from build123d import *

# Parameters (mm, degrees)
SKETCH1_R           = 40
BOSS_EXTRUDE1_DEPTH = 4
SKETCH2_R           = 25
BOSS_EXTRUDE2_DEPTH = 6
SKETCH3_R           = 1.5
CUT_EXTRUDE1_DEPTH  = 5
SKETCH4_R           = 9
CUT_EXTRUDE2_DEPTH  = 58.445626465
SKETCH5_R           = 1.5
CUT_EXTRUDE3_DEPTH  = 57.789083458
SKETCH6_R           = 2.84
CUT_EXTRUDE4_DEPTH  = 3


with BuildPart() as part:
    # Sketch1 → Boss-Extrude1 (new body)
    with BuildSketch(Plane(origin=(0, 0, 0), x_dir=(1, 0, 0), z_dir=(0, 1, 0))):
        with Locations(Location((0, 0, 0), (0, 0, 270))):
            Circle(SKETCH1_R)
    extrude(amount=BOSS_EXTRUDE1_DEPTH)

    # Sketch2 → Boss-Extrude2 (add)
    with BuildSketch(Plane(origin=(0, 4, 0), x_dir=(1, 0, 0), z_dir=(0, 1, 0))):
        with Locations(Location((0, 0, 0), (0, 0, 270))):
            Circle(SKETCH2_R)
    extrude(amount=BOSS_EXTRUDE2_DEPTH)

    # Sketch3 → Cut-Extrude1 (cut)
    with BuildSketch(Plane(origin=(0, 10, 0), x_dir=(1, 0, 0), z_dir=(0, 1, 0))):
        with Locations(Location((0, -21.5, 0), (0, 0, 270))):
            Circle(SKETCH3_R)
        with Locations(Location((-15.202795796, -15.202795796, 0), (0, 0, 270))):
            Circle(SKETCH3_R)
        with Locations(Location((-21.5, 0, 0), (0, 0, 270))):
            Circle(SKETCH3_R)
        with Locations(Location((-15.202795796, 15.202795796, 0), (0, 0, 270))):
            Circle(SKETCH3_R)
        with Locations(Location((0, 21.5, 0), (0, 0, 270))):
            Circle(SKETCH3_R)
        with Locations(Location((15.202795796, 15.202795796, 0), (0, 0, 270))):
            Circle(SKETCH3_R)
        with Locations(Location((21.5, 0, 0), (0, 0, 270))):
            Circle(SKETCH3_R)
        with Locations(Location((15.202795796, -15.202795796, 0), (0, 0, 270))):
            Circle(SKETCH3_R)
    extrude(amount=-CUT_EXTRUDE1_DEPTH, mode=Mode.SUBTRACT)

    # Sketch4 → Cut-Extrude2 (cut, through all)
    with BuildSketch(Plane(origin=(0, 10, 0), x_dir=(1, 0, 0), z_dir=(0, 1, 0))):
        with Locations(Location((0, 0, 0), (0, 0, 270))):
            Circle(SKETCH4_R)
    extrude(amount=-CUT_EXTRUDE2_DEPTH, mode=Mode.SUBTRACT)

    # Sketch5 → Cut-Extrude3 (cut, through all)
    with BuildSketch(Plane(origin=(0, 5, 0), x_dir=(1, 0, 0), z_dir=(0, 1, 0))):
        with Locations(Location((15.202795796, 15.202795796, 0), (0, 0, 270))):
            Circle(SKETCH5_R)
        with Locations(Location((-15.202795796, -15.202795796, 0), (0, 0, 270))):
            Circle(SKETCH5_R)
    extrude(amount=-CUT_EXTRUDE3_DEPTH, mode=Mode.SUBTRACT)

    # Sketch6 → Cut-Extrude4 (cut)
    with BuildSketch(Plane.XZ):
        with Locations(Location((-15.202795796, 15.202795796, 0), (0, 0, 270))):
            Circle(SKETCH6_R)
        with Locations(Location((15.202795796, -15.202795796, 0), (0, 0, 270))):
            Circle(SKETCH6_R)
    extrude(amount=-CUT_EXTRUDE4_DEPTH, mode=Mode.SUBTRACT)


solid = part.part
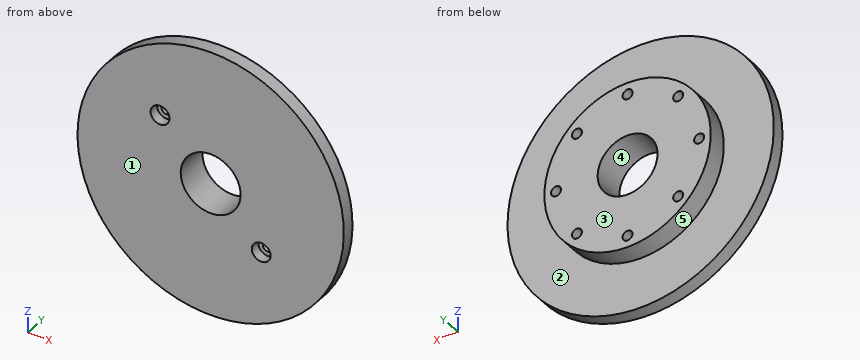
Here's how the part is built. I have some questions about the finished solid (model axes, mm). Face numbers are marked on the shaded views. A direction names the side the tool comes from. Round coordinates to 2 decimals unless told otherwise and drop trailing zeros. Write each loop counter-clockwise with the first axis right and the second up, starting at its lowest first coordinate (ties: lowest second). Pieces come first, ordered by that corner, then holes.
1. Will these pins go through, and if not, where does the flat tip stop? pin 1 Ø1.5 at (y, z) = (4, -3) entering from -X; pin 2 Ø5 at (y, z) = (4, 1) entering from -X; pin 3 Ø1.5 at (x, z) = (0.5, -21.5) entering from +Y.
2. For the marked faces 1 and 2, which set-ups out of +Z, -Z, +X, -X, +Y, -Y let a thin tool reach every point of the face, with its end or its side?
3. If we mould it in two halves opening along X, with no side actions, what happens to the marked faces 3, 4 and 5? For each: released by +X, released by -X, zero draft, split by the parting line, or undercut.
4. I need wall thicknesses on L1, parallel to Y at x = -10, z = -26.5; L2, parallel to Z at x = -8, y = 6.25; L3, parallel to Z at x = -4.5, y = 5.25. Which ranges of each line are inside material? Lowest first, please.
5. Suppose I cut it at B-B (z = -6.5). List the corners of the cut face in (x, y) for me.
6. Suppose I cut it at C-C (y = 8). State how many separate pieces and enclosed holes the cut face has, and give its area (3 significant figures).
7. Suppose I cut it at A-A (x = 0). List the corners of the cut face in (y, z) for me.
8. Suppose I cut it at D-D (x = 19). List the corners of the cut face in (y, z) for me.
Answer sheet:
1. pin 1: stops at x = -39.94
1. pin 2: stops at x = -40
1. pin 3: stops at y = 5
2. face 1: +Z, -Z, +X, -X, -Y
2. face 2: +Y
3. face 3: zero draft
3. face 4: undercut
3. face 5: split by the parting line
4. L1: y = 0 to 4
4. L2: z = -23.69 to -4.12, 4.12 to 23.69
4. L3: z = -24.59 to -7.79, 7.79 to 24.59
5. outline: (-39.47, 0) - (-6.22, 0) - (-6.22, 10) - (-24.14, 10) - (-24.14, 4) - (-39.47, 4) - close; (6.22, 0) - (39.47, 0) - (39.47, 4) - (24.14, 4) - (24.14, 10) - (6.22, 10) - close
6. separate pieces: 1
6. enclosed holes: 9
6. area: 1,650 mm2
7. outline: (0, -40) - (4, -40) - (4, -25) - (10, -25) - (10, -23) - (5, -23) - (5, -20) - (10, -20) - (10, -9) - (0, -9) - close; (0, 9) - (10, 9) - (10, 20) - (5, 20) - (5, 23) - (10, 23) - (10, 25) - (4, 25) - (4, 40) - (0, 40) - close
8. outline: (0, -35.2) - (4, -35.2) - (4, -16.25) - (10, -16.25) - (10, 16.25) - (4, 16.25) - (4, 35.2) - (0, 35.2) - close
